Design review of the part built by this model. Coordinates are the model's own, in mm. Face numbers are marked on the shaded views. A direction names the side the tool comes from. Round coordinates to 2 decimals unless told otherwise and drop trailing zeros. Write each loop counter-clockwise with the first axis right and the second up, starting at its lowest first coordinate (ties: lowest second). Pieces come first, ordered by that corner, then holes. Notation, with made-up numbers: (10.25, -25) -> (31.25, -25) arc R6 cw to (31.25, -14) -> close; hole circle Ø10 at (-4, 38.5). An arc over 180 degrees is marked (long way). One line per question, with ' | ' between items. Start each with the question number.
1) Consider section B-B (y = 14.5). Give the boundary of the cut face in (x, z) (3 decimals).
2) For probe 1 along X at (y, z) = (1.25, 0) (3 decimals); probe 2 along X at (y, z) = (13.5, 2.75); probe 3 along Z at (x, y) = (-0.5, 15), list the stretches that pass through material, from the lowest coordinate up.
3) Insertion check: pin 1 Ø0.9 at (y, z) = (12, 0) entering from +X (3 decimals); pin 2 Ø3.5 at (x, z) = (1, -0.5) entering from +Y; pin 3 Ø2 at (x, y) = (2.5, 3.5) entering from -Z. Each pin has a flat end and moves straight along its axis. Give the tip position at first contact, or say it passes through.
4) Consider section C-C (y = 1.5). Give the boundary of the cut face in (x, z) (3 decimals), then the cut area to 3 significant figures.
5) Consider section D-D (z = 4). Give the boundary of the cut face in (x, y).
6) Mouldability with a two-part tool opening along X and no side actions: class the marked faces 1, 2 and 3 as +X half, -X half, draft (parallel to the pull), parting line (faces both ways), or undercut.
7) For the marked faces 4 and 5, list the 3-axis set-ups (+Z, -Z, +X, -X, +Y, -Y) from which the entire face can be reached by the end or side of a thin tool; tool diameter is ignored.
8) Consider section A-A (z = 0). Give the boundary of the cut face in (x, y) (3 decimals), then the cut area to 3 significant figures.
```python
from build123d import *

# Parameters (mm, degrees)
SKETCH1_R           = 7
BOSS_EXTRUDE1_DEPTH = 10
SKETCH2_R           = 5.075
BOSS_EXTRUDE2_DEPTH = 6
CUT_EXTRUDE2_DEPTH  = 19.814887722
SKETCH5_OUTSIDE_W   = 21.092
SKETCH5_OUTSIDE_H   = 21.092
SKETCH5_OUTSIDE_R   = 5.5
CUT_EXTRUDE3_DEPTH  = 15.071247279


with BuildPart() as part:
    # Sketch1 → Boss-Extrude1 (new body)
    with BuildSketch(Plane(origin=(0, 0, 0), x_dir=(1, 0, 0), z_dir=(0, 1, 0))):
        with Locations(Location((0, 0, 0), (0, 0, 270))):
            Circle(SKETCH1_R)
    extrude(amount=BOSS_EXTRUDE1_DEPTH)

    # Sketch2 → Boss-Extrude2 (add)
    with BuildSketch(Plane(origin=(0, 10, 0), x_dir=(1, 0, 0), z_dir=(0, 1, 0))):
        with Locations(Location((0, 0, 0), (0, 0, 270))):
            Circle(SKETCH2_R)
    extrude(amount=BOSS_EXTRUDE2_DEPTH)

    # Sketch4 → Cut-Extrude2 (cut, through all)
    with BuildSketch(Plane(origin=(0, 16, 0), x_dir=(1, 0, 0), z_dir=(0, 1, 0))):
        Polygon((2.525, 1.45780943), (0, 2.915618859), (-2.525, 1.45780943), (-2.525, -1.45780943), (0, -2.915618859), (2.525, -1.45780943), align=None)
    extrude(amount=-CUT_EXTRUDE2_DEPTH, mode=Mode.SUBTRACT)

    # Sketch5 outside → Cut-Extrude3 (cut, through all)
    with BuildSketch(Plane(origin=(0, 10, 0), x_dir=(1, 0, 0), z_dir=(0, 1, 0))):
        Rectangle(SKETCH5_OUTSIDE_W, SKETCH5_OUTSIDE_H)
        with Locations(Location((0, 0, 0), (0, 0, 270))):
            Circle(SKETCH5_OUTSIDE_R, mode=Mode.SUBTRACT)
    extrude(amount=-CUT_EXTRUDE3_DEPTH, mode=Mode.SUBTRACT)


solid = part.part
```
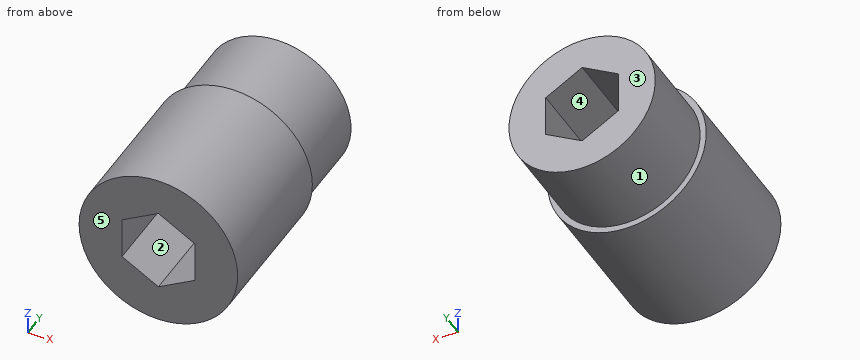
From the geometry:
1) outline: circle Ø10.15 at (0, 0); hole (-2.525, -1.458) -> (0, -2.916) -> (2.525, -1.458) -> (2.525, 1.458) -> (0, 2.916) -> (-2.525, 1.458) -> close
2) probe 1: x = -5.5 to -2.525, 2.525 to 5.5 | probe 2: x = -4.27 to -0.29, 0.29 to 4.27 | probe 3: z = -5.05 to -2.63, 2.63 to 5.05
3) pin 1: stops at x = 5.075 | pin 2: stops at y = 16 | pin 3: stops at z = -5.29
4) outline: circle Ø11 at (0, 0); hole (-2.525, -1.458) -> (0, -2.916) -> (2.525, -1.458) -> (2.525, 1.458) -> (0, 2.916) -> (-2.525, 1.458) -> close | area: 72.9 mm2
5) outline: (-3.77, 0) -> (3.77, 0) -> (3.77, 10) -> (3.12, 10) -> (3.12, 16) -> (-3.12, 16) -> (-3.12, 10) -> (-3.77, 10) -> close
6) face 1: parting line | face 2: undercut | face 3: draft
7) face 4: +Y, -Y | face 5: +Z, -Z, +X, -X, -Y
8) outline: (-5.5, 0) -> (-2.525, 0) -> (-2.525, 16) -> (-5.075, 16) -> (-5.075, 10) -> (-5.5, 10) -> close; (2.525, 0) -> (5.5, 0) -> (5.5, 10) -> (5.075, 10) -> (5.075, 16) -> (2.525, 16) -> close | area: 90.1 mm2
